from build123d import *

# Parameters (mm, degrees)
EXTRUDE_4_DEPTH          = 10
SKETCH_5_R               = 2
CUT_EXTRUDE_3_DEPTH      = 252.035308536
PATTERN_CIRCULAR_1_COUNT = 6
SKETCH_6_R               = 3.5
CUT_EXTRUDE_4_DEPTH      = 252.035308536
PATTERN_CIRCULAR_2_COUNT = 6
SKETCH_7_R               = 7
CUT_EXTRUDE_6_DEPTH      = 252.035308536
SKETCH_11_R              = 4.5
EXTRUDE_5_DEPTH          = 10
PATTERN_CIRCULAR_3_COUNT = 6
SKETCH_15_R              = 10
EXTRUDE_6_DEPTH          = 10
SKETCH_26_R              = 50
EXTRUDE_10_DEPTH         = 5
SKETCH_26_5_OUTSIDE_W    = 174.739
SKETCH_26_5_OUTSIDE_H    = 341.75
SKETCH_26_5_OUTSIDE_R    = 50
SKETCH_26_5_OUTSIDE_R_2  = 2
CUT_EXTRUDE_14_DEPTH     = 5
SKETCH_27_R              = 50
EXTRUDE_11_DEPTH         = 65
CUT_EXTRUDE_START        = -5
CUT_EXTRUDE_16_DEPTH     = 55
CUT_EXTRUDE_START_2      = -60
CUT_EXTRUDE_18_DEPTH     = 55
SKETCH_31_R              = 1.75
CUT_EXTRUDE_19_DEPTH     = 5
PATTERN_CIRCULAR_4_COUNT = 8
SKETCH_32_R              = 9
SKETCH_32_R_2            = 7
EXTRUDE_12_DEPTH         = 2
SKETCH_33_R              = 3
CUT_EXTRUDE_20_DEPTH     = 271.034675795
SKETCH_34_R              = 4
CUT_EXTRUDE_21_DEPTH     = 10


with BuildPart() as part:
    # Sketch 2 → Extrude 4 (new body)
    with BuildSketch(Plane(origin=(0, 0, 0), x_dir=(1, 0, 0), z_dir=(0, 1, 0))):
        with BuildLine():
            Line((0, 0), (0, -32))
            Line((0, -32), (51.194707256, -155.834978697))
            Line((51.194707256, -155.834978697), (51.194707256, -195.834978697))
            ThreePointArc((51.194707256, -195.834978697), (80.694707256, -225.334978697), (110.194707256, -195.834978697))
            Line((110.194707256, -195.834978697), (110.194707256, -163.834978697))
            Line((110.194707256, -163.834978697), (76.523567349, -58.065160992))
            Line((76.523567349, -58.065160992), (96.300654989, 2.802456051))
            ThreePointArc((96.300654989, 2.802456051), (46.666363617, 52.394603419), (0, 0))
        make_face()
    extrude(amount=EXTRUDE_4_DEPTH)

    # Sketch 5 → Cut-Extrude 3 (cut, through all)
    with BuildSketch(Plane(origin=(0, 10, 0), x_dir=(1, 0, 0), z_dir=(0, 1, 0))):
        with Locations(Location((48.06989804, 16.403739233, 0), (0, 0, 270))):
            Circle(SKETCH_5_R)
    cut_extrude_3 = extrude(amount=-CUT_EXTRUDE_3_DEPTH, mode=Mode.SUBTRACT)

    # Pattern Circular 1: Cut-Extrude 3 ×6 about axis
    pattern_circular_1_axis = Axis((48.06989804, 0, -4.165021303), (0, 1, 0))
    for i in range(1, PATTERN_CIRCULAR_1_COUNT):
        add(cut_extrude_3.rotate(pattern_circular_1_axis, i * 360 / PATTERN_CIRCULAR_1_COUNT), mode=Mode.SUBTRACT)

    # Sketch 6 → Cut-Extrude 4 (cut, through all)
    with BuildSketch(Plane(origin=(0, 10, 0), x_dir=(1, 0, 0), z_dir=(0, 1, 0))):
        with Locations(Location((9.773410956, 4.165021303, 0), (0, 0, 270))):
            Circle(SKETCH_6_R)
    cut_extrude_4 = extrude(amount=-CUT_EXTRUDE_4_DEPTH, mode=Mode.SUBTRACT)

    # Pattern Circular 2: Cut-Extrude 4 ×6 about axis
    pattern_circular_2_axis = Axis((48.06989804, 0, -4.165021303), (0, 1, 0))
    for i in range(1, PATTERN_CIRCULAR_2_COUNT):
        add(cut_extrude_4.rotate(pattern_circular_2_axis, i * 360 / PATTERN_CIRCULAR_2_COUNT), mode=Mode.SUBTRACT)

    # Sketch 7 → Cut-Extrude 6 (cut, through all)
    with BuildSketch(Plane(origin=(0, 10, 0), x_dir=(1, 0, 0), z_dir=(0, 1, 0))):
        with Locations(Location((80.694707256, -208.084978697, 0), (0, 0, 270))):
            Circle(SKETCH_7_R)
    extrude(amount=-CUT_EXTRUDE_6_DEPTH, mode=Mode.SUBTRACT)


with BuildPart() as body_2:
    # Mirror 6: mirrored copy
    add(part.part.mirror(Plane.ZX.offset(-5)))


with BuildPart() as part_1:
    add(part.part)

    add(body_2.part)  # Extrude 5 merges body 2
    # Sketch 11 → Extrude 5 (add, symmetric)
    with BuildSketch(Plane(origin=(0, -5, 0), x_dir=(1, 0, 0), z_dir=(0, 1, 0))):
        with Locations(Location((9.773410956, 4.165021303, 0), (0, 0, 90))):
            Circle(SKETCH_11_R)
    extrude_5 = extrude(amount=EXTRUDE_5_DEPTH, both=True)

    # Pattern Circular 3: Extrude 5 ×6 about axis
    pattern_circular_3_axis = Axis((48.06989804, 0, -4.165021303), (0, 1, 0))
    for i in range(1, PATTERN_CIRCULAR_3_COUNT):
        add(extrude_5.rotate(pattern_circular_3_axis, i * 360 / PATTERN_CIRCULAR_3_COUNT))

    # Sketch 15 → Extrude 6 (add)
    with BuildSketch(Plane(origin=(0, -10, 0), x_dir=(1, 0, 0), z_dir=(0, 1, 0))):
        with Locations(Location((40.25784211, -76.11542009, 0), (0, 0, 270))):
            Circle(SKETCH_15_R)
        with Locations(Location((59.742285998, -134.794304017, 0), (0, 0, 270))):
            Circle(SKETCH_15_R)
    extrude(amount=EXTRUDE_6_DEPTH)

    # Sketch 26 → Extrude 10 (add)
    with BuildSketch(Plane(origin=(0, -20, 0), x_dir=(-1, 0, 0), z_dir=(0, -1, 0))):
        with Locations(Location((-48.034216366, 3.837134188, 0), (0, 0, 220.410394995))):
            Circle(SKETCH_26_R)
    extrude(amount=EXTRUDE_10_DEPTH)

    # Sketch 26_5 outside → Cut-Extrude 14 (cut)
    # profile 1 of 7: a face of its own
    with BuildSketch(Plane(origin=(0, -20, 0), x_dir=(-1, 0, 0), z_dir=(0, -1, 0))):
        with Locations((-54.1145, -85.749)):
            Rectangle(SKETCH_26_5_OUTSIDE_W, SKETCH_26_5_OUTSIDE_H)
        with Locations(Location((-48.034216366, 3.837134188, 0), (0, 0, 220.410394995))):
            Circle(SKETCH_26_5_OUTSIDE_R, mode=Mode.SUBTRACT)
    # profile 2 of 7: a face of its own
    with BuildSketch(Plane(origin=(0, -20, 0), x_dir=(-1, 0, 0), z_dir=(0, -1, 0))):
        with Locations(Location((-48.06989804, 16.403739233, 0), (0, 0, 270))):
            Circle(SKETCH_26_5_OUTSIDE_R_2)
    # profile 3 of 7: a face of its own
    with BuildSketch(Plane(origin=(0, -20, 0), x_dir=(-1, 0, 0), z_dir=(0, -1, 0))):
        with Locations(Location((-37.470857403, 10.284380268, 0), (0, 0, 210))):
            Circle(SKETCH_26_5_OUTSIDE_R_2)
    # profile 4 of 7: a face of its own
    with BuildSketch(Plane(origin=(0, -20, 0), x_dir=(-1, 0, 0), z_dir=(0, -1, 0))):
        with Locations(Location((-37.470857403, -1.954337662, 0), (0, 0, 150))):
            Circle(SKETCH_26_5_OUTSIDE_R_2)
    # profile 5 of 7: a face of its own
    with BuildSketch(Plane(origin=(0, -20, 0), x_dir=(-1, 0, 0), z_dir=(0, -1, 0))):
        with Locations(Location((-48.06989804, -8.073696627, 0), (0, 0, 90))):
            Circle(SKETCH_26_5_OUTSIDE_R_2)
    # profile 6 of 7: a face of its own
    with BuildSketch(Plane(origin=(0, -20, 0), x_dir=(-1, 0, 0), z_dir=(0, -1, 0))):
        with Locations(Location((-58.668938677, -1.954337662, 0), (0, 0, 30))):
            Circle(SKETCH_26_5_OUTSIDE_R_2)
    # profile 7 of 7: a face of its own
    with BuildSketch(Plane(origin=(0, -20, 0), x_dir=(-1, 0, 0), z_dir=(0, -1, 0))):
        with Locations(Location((-58.668938677, 10.284380268, 0), (0, 0, 330))):
            Circle(SKETCH_26_5_OUTSIDE_R_2)
    extrude(amount=CUT_EXTRUDE_14_DEPTH, mode=Mode.SUBTRACT)

    # Sketch 27 → Extrude 11 (add)
    with BuildSketch(Plane.XZ.offset(25)):
        with Locations(Location((48.034216366, -3.837134188, 0), (0, 0, 40.410394995))):
            Circle(SKETCH_27_R)
    extrude(amount=EXTRUDE_11_DEPTH)

    # Sketch 30 → Cut-Extrude 16 (cut)
    with BuildSketch(Plane.XZ.offset(90).offset(CUT_EXTRUDE_START)):
        with BuildLine():
            Line((0, 0), (95.845046759, 0))
            ThreePointArc((95.845046759, 0), (47.922523379, -52.010409834), (0, 0))
        make_face()
    extrude(amount=-CUT_EXTRUDE_16_DEPTH, mode=Mode.SUBTRACT)

    # Sketch 28 → Cut-Extrude 18 (cut)
    with BuildSketch(Plane.XZ.offset(90).offset(CUT_EXTRUDE_START_2)):
        with BuildLine():
            Line((-1.818330221, 0), (97.886762953, 0))
            ThreePointArc((97.886762953, 0), (48.034216366, 46.162865812), (-1.818330221, 0))
        make_face()
    extrude(amount=CUT_EXTRUDE_18_DEPTH, mode=Mode.SUBTRACT)

    # Sketch 31 → Cut-Extrude 19 (cut)
    with BuildSketch(Plane(origin=(0, -90, 0), x_dir=(-1, 0, 0), z_dir=(0, -1, 0))):
        with Locations(Location((-48.034216366, 46.337134188, 0), (0, 0, 90))):
            Circle(SKETCH_31_R)
    cut_extrude_19 = extrude(amount=-CUT_EXTRUDE_19_DEPTH, mode=Mode.SUBTRACT)

    # Pattern Circular 4: Cut-Extrude 19 ×8 about axis
    pattern_circular_4_axis = Axis((48.034216366, 0, -3.837134188), (0, 1, 0))
    for i in range(1, PATTERN_CIRCULAR_4_COUNT):
        add(cut_extrude_19.rotate(pattern_circular_4_axis, i * 360 / PATTERN_CIRCULAR_4_COUNT), mode=Mode.SUBTRACT)

    # Sketch 32 → Extrude 12 (add)
    with BuildSketch(Plane.XZ.offset(20)):
        with Locations(Location((80.694707256, 208.084978697, 0), (0, 0, 90))):
            Circle(SKETCH_32_R)
        with Locations(Location((80.694707256, 208.084978697, 0), (0, 0, 90))):
            Circle(SKETCH_32_R_2, mode=Mode.SUBTRACT)
    extrude_12 = extrude(amount=EXTRUDE_12_DEPTH)

    # Sketch 33 → Cut-Extrude 20 (cut, through all)
    with BuildSketch(Plane(origin=(0, 10, 0), x_dir=(1, 0, 0), z_dir=(0, 1, 0))):
        with Locations(Location((68.993287967, -71.793228779, 0), (0, 0, 270))):
            Circle(SKETCH_33_R)
        with Locations(Location((76.658249851, -93.478439392, 0), (0, 0, 270))):
            Circle(SKETCH_33_R)
        with Locations(Location((83.323434097, -112.335144272, 0), (0, 0, 270))):
            Circle(SKETCH_33_R)
        with Locations(Location((89.988618344, -131.191849153, 0), (0, 0, 270))):
            Circle(SKETCH_33_R)
    extrude(amount=-CUT_EXTRUDE_20_DEPTH, mode=Mode.SUBTRACT)

    # Sketch 34 → Cut-Extrude 21 (cut)
    with BuildSketch(Plane(origin=(0, 10, 0), x_dir=(1, 0, 0), z_dir=(0, 1, 0))):
        with Locations(Location((35.681581865, -77.846678561, 0), (0, 0, 270))):
            Circle(SKETCH_34_R)
        with Locations(Location((41.53805169, -110.53992851, 0), (0, 0, 270))):
            Circle(SKETCH_34_R)
        with Locations(Location((60.383294084, -136.076495377, 0), (0, 0, 270))):
            Circle(SKETCH_34_R)
    cut_extrude_21 = extrude(amount=-CUT_EXTRUDE_21_DEPTH, mode=Mode.SUBTRACT)

    # Mirror 7: Cut-Extrude 21 across plane
    add(cut_extrude_21.mirror(Plane.ZX.offset(-5)), mode=Mode.SUBTRACT)

    # Mirror 8: Extrude 12 across plane
    add(extrude_12.mirror(Plane.ZX.offset(-5)))


solid = part_1.part
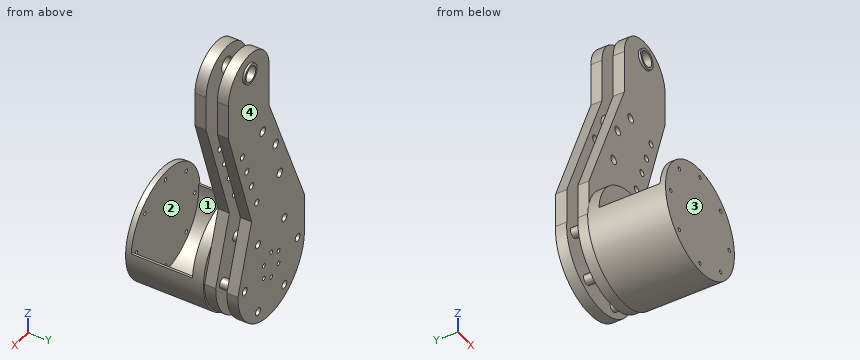
Input: part model. Units: mm. Frame: model coordinates. Face numbers are marked on the shaded views. Round coordinates to 2 decimals unless told otherwise and drop trailing zeros. Order: outer loops, then holes, each group sorted by start corner. A loop starts at its lowest first (then second) coordinate and runs counter-clockwise, first axis right, second up. Notation, with made-up numbers: (-22.75, 41) - (1.25, 41) arc R20 cw to (1.25, 58) - close; hole circle Ø9 at (42.5, 17). An arc over 180 degrees is marked (long way). Answer as a JSON object with one key per item and string values. Group by question number.
(1) Cut plane B-B (y = -4). Return loops of the section in (x, z).
(2) Draft query along Y for the marked faces 1, 2, 3 and 4. Return one class per face: released by +Y, released by -Y, zero draft, split by the parting line, or undercut.
(3) Cut plane A-A (z = 55). Return loops of the section in (x, y), then the cut area to 3 significant figures.
(4) Cut plane D-D (y = -43). Return loops of the section in (x, z), then the cut area to 3 significant figures.
(5) Cut plane C-C (z = 119). Return loops of the section in (x, y).
(6) Material intervals for probe 1 along Y at (x, z) = (62.5, 38.5); probe 2 along Y at (x, z) = (39, 122); probe 3 along Z at (x, y) = (82.5, -49), sorted ascending. Write a range as from..to.
(7) Pin query (flat end, axial travel): P1, Ø9.5, axis at x = 68.99, z = 71.79, coming from the +Y side; P2, Ø6, axis at x = 43, y = -24, coming from the -Z side; P3, Ø1.5, axis at x = 71, z = 137.5, coming from the -Y side; P4, Ø3.5, axis at x = 76.66, z = 93.48, coming from the -Y side. Return the tip coordinate at first contact, or that it passes through.
Here are the results:
{
 "1": {"outline": "circle Ø9 at (9.77, -4.17); circle Ø9 at (28.92, -37.33); circle Ø9 at (28.92, 29); circle Ø20 at (40.26, 76.12); circle Ø20 at (59.74, 134.79); circle Ø9 at (67.22, -37.33); circle Ø9 at (67.22, 29); circle Ø9 at (86.37, -4.17)"},
 "2": {"face 1": "undercut", "face 2": "undercut", "face 3": "released by -Y", "face 4": "released by +Y"},
 "3": {"outline": "(9.51, -20) - (77.52, -20) - (77.52, -10) - (9.51, -10) - close; (9.51, 0) - (77.52, 0) - (77.52, 10) - (9.51, 10) - close", "area": "1,360 mm^2"},
 "4": {"outline": "(-1.82, 0) arc R50 ccw (long way) to (97.89, 0) - (95.85, 0) arc R48.08 cw (long way) to (0, 0) - close", "area": "301 mm^2"},
 "5": {"outline": "(35.97, -20) - (95.92, -20) - (95.92, -10) - (35.97, -10) - close; (35.97, 0) - (95.92, 0) - (95.92, 10) - (35.97, 10) - close"},
 "6": {"probe 1": "y = -90..-85, -30..-10, 0..10", "probe 2": "y = -20..-10, 0..10", "probe 3": "z = -40.06..-37.34"},
 "7": {"P1": "stops at y = 10", "P2": "stops at z = -53.8", "P3": "stops at y = -20", "P4": "passes through"}
}
